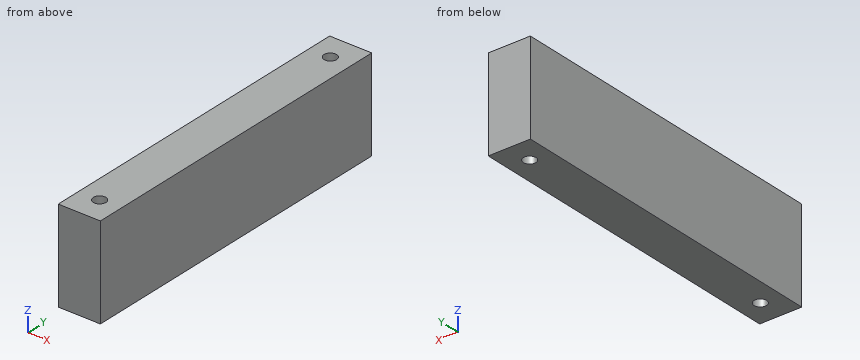
Autodesk Inventor part; units mm, degrees
ref_plane "YZ Plane" through (0, 0, 0) normal (1, 0, 0) x (0, 1, 0)
ref_plane "XZ Plane" through (0, 0, 0) normal (0, 1, 0) x (-1, 0, 0)
ref_plane "XY Plane" through (0, 0, 0) normal (0, 0, 1) x (1, 0, 0)
sketch "Boceto1" plane through (0, 0, 0) normal (0, 1, 0) x (-1, 0, 0)
  line L0 (-25, 55) -> (25, 55)
  line L1 (25, 55) -> (25, -55)
  line L2 (25, -55) -> (-25, -55)
  line L3 (-25, -55) -> (-25, 55)
  line L4 (-25, 55) -> (25, -55) construction
  line L5 (25, 55) -> (-25, -55) construction
  point P0 (0, 0)
  dimension "d0" = 50
  dimension "d1" = 110
extrude "Extrusión1" add sketch "Boceto1" along normal blind 400
sketch "Boceto2" plane through (-25, 0, 55) normal (0, 0, 1) x (1, 0, 0)
  line L0 (0, 400) -> (50, 400)
  line L1 (25, 400) -> (25, 370)
  line L2 (25, 0) -> (25, 30)
  circle A0 centre (25, 370) radius 7.5
  circle A1 centre (25, 30) radius 7.5
  dimension "d4" = 30
  dimension "d5" = 30
  dimension "d6" = 15
  dimension "d7" = 15
extrude "Extrusión2" cut sketch "Boceto2" against normal up to next
properties part number "brazo2"
Design review of the part built by this model. Coordinates are the model's own, in mm. Give positions to 0.01 mm unless a question says otherwise; leave off trailing zeros. Order: outer loops, then holes, each group sorted by start corner. A loop starts at its lowest first (then second) coordinate and runs counter-clockwise, first axis right, second up. Notation, with made-up numbers: M 62.5,-27.75 L 90.5,-27.75 A26 cw 90.5,10.25 Z; hole C -12,47 d5. An arc over 180 degrees is marked long. One line per question, with ' | ' between items. Start each with the question number.
Q1. We need section C-C (z = -21.5). Write out the cut boundary in (x, y).
Q2. We need section B-B (y = 30). Write out the cut boundary in (x, z), plus the area to 3 significant figures.
Q3. For pin 1 Ø12 at (x, y) = (0, 30) entering from +Z, flat-tipped, find the tip position at first contact; note if it passes through.
Q4. We need section A-A (x = 0). Write out the cut boundary in (y, z), plus the area to 3 significant figures.
Q5. For L1, parallel to Y at x = 0, z = 7; L2, parallel to X at y = 370, z = -2; L3, parallel to Y at x = 4, z = 17, list the stretches that pass through material, from the lowest coordinate up. Write a range as [from, to].
Returned:
1) outline: M -25,0 L 25,0 L 25,400 L -25,400 Z; hole C 0,30 d15; hole C 0,370 d15
2) outline: M -25,-55 L -7.5,-55 L -7.5,55 L -25,55 Z; M 7.5,-55 L 25,-55 L 25,55 L 7.5,55 Z | area: 3,850 mm2
3) pin 1: through
4) outline: M 0,-55 L 22.5,-55 L 22.5,55 L 0,55 Z; M 37.5,-55 L 362.5,-55 L 362.5,55 L 37.5,55 Z; M 377.5,-55 L 400,-55 L 400,55 L 377.5,55 Z | area: 40,700 mm2
5) L1: [0, 22.5], [37.5, 362.5], [377.5, 400] | L2: [-25, -7.5], [7.5, 25] | L3: [0, 23.66], [36.34, 363.66], [376.34, 400]
